For this review, use the dimensioned drawing (mm, ordinates from the lowest corner) and the shaded views. A direction names the side the tool comes from. Give positions to 0.01 mm unless a question says otherwise; leave off trailing zeros. Loops run counter-clockwise (first coordinate to the right, second up) from the corner with the lowest first, then second, coordinate; pieces in that order, holes last. Notation, with made-up numbers: M 35,4.25 L 55,4.25 A10 cw 55,15.25 Z; hole C 48,-19.5 d10. An arc over 180 degrees is marked long. Use a Markdown table: item, result. Add a question column.
(1) Add section C-C, the plane y = 28. Give the boundary of the cut face in (x, z).
(2) Add section A-A, the plane x = 7. Give the boundary of the cut face in (y, z), then the cut area to 3 significant figures.
(3) Add section B-B, the plane z = 5.75. Give the boundary of the cut face in (x, y).
(4) Add section D-D, the plane x = 11.75. Give the boundary of the cut face in (y, z).
(5) Insertion check: pin 1 Ø2 at (x, y) = (8.5, 17.5) entering from -Z; pin 2 Ø4 at (x, y) = (2, 14.5) entering from -Z; pin 3 Ø6.5 at (x, z) = (9, 3.5) entering from -Y. Each pin has a flat end and moves straight along its axis. Give the tip position at first contact, or say it passes through.
(6) For the marked faces 1, 2 and 3, list the 3-axis set-ups (+Z, -Z, +X, -X, +Y, -Y) from which the entire face can be reached by the end or side of a thin tool; tool diameter is ignored.
(7) For probe 1 along Z at (x, y) = (8.75, 6); probe 2 along Y at (x, z) = (1.5, 4.5); probe 3 along X at (y, z) = (29, 8.5), list the stretches that pass through material, from the lowest coordinate up.
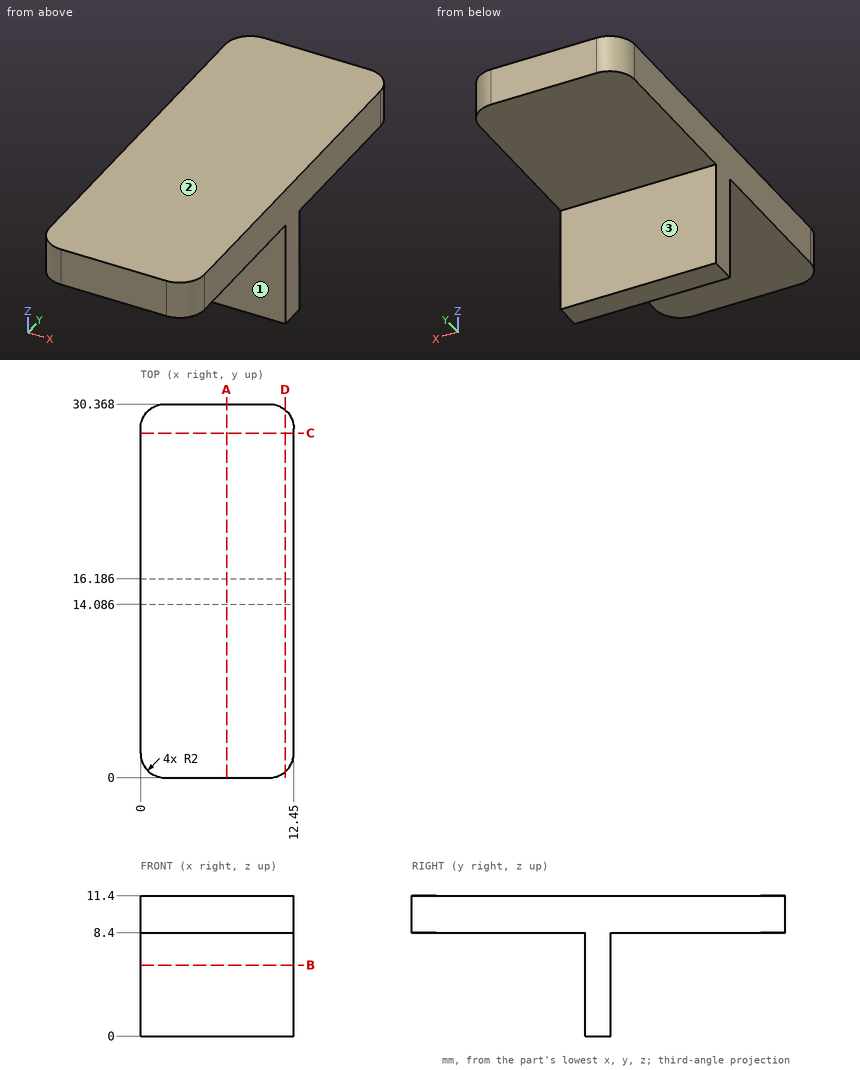
Established:
| question | item | result |
|---|---|---|
| 1 | outline | M 0,8.4 L 12.45,8.4 L 12.45,11.4 L 0,11.4 Z |
| 2 | outline | M 0,8.4 L 14.09,8.4 L 14.09,0 L 16.19,0 L 16.19,8.4 L 30.37,8.4 L 30.37,11.4 L 0,11.4 Z |
| 2 | area | 109 mm^2 |
| 3 | outline | M 0,14.09 L 12.45,14.09 L 12.45,16.19 L 0,16.19 Z |
| 4 | outline | M 0.48,8.4 L 14.09,8.4 L 14.09,0 L 16.19,0 L 16.19,8.4 L 29.89,8.4 L 29.89,11.4 L 0.48,11.4 Z |
| 5 | pin 1 | z = 8.4 |
| 5 | pin 2 | z = 0 |
| 5 | pin 3 | y = 14.09 |
| 6 | face 1 | -Z, +X, -X, -Y |
| 6 | face 2 | +Z, +X, -X, +Y, -Y |
| 6 | face 3 | -Z, +X, -X, +Y |
| 7 | probe 1 | 8.4 to 11.4 |
| 7 | probe 2 | 14.09 to 16.19 |
| 7 | probe 3 | 0.1 to 12.35 |
